Work out the finished part from the listing and answer in its coordinate system (mm). A direction names the side the tool comes from. Coordinates: 2 decimals unless noted, no trailing zeros. Loops run counter-clockwise (first coordinate to the right, second up) from the corner with the lowest first, then second, coordinate; pieces in that order, holes last. Notation, with made-up numbers: (65.25, 59) - (81.25, 59) arc R36 ccw to (81.25, 97) - close; hole circle Ø11 at (53, 28.5). An arc over 180 degrees is marked (long way). Write each question's results on one line, items separated by ' | '. Start each with the question number.
1. A cutting plane is placed at B-B on x = 0. Determine the outline of the cut face in (y, z), then the cut area to 3 significant figures.
2. A cutting plane is placed at C-C on z = 37.5. Determine the outline of the cut face in (x, y).
3. Determine the mould class of faces 1 (the cylindrical face through (-1.319, -7.395, -59.985)), 2 (the cylindrical face through (-2.17, -7.4, 20.24)), 3 (the cylindrical face through (-2.17, -7.4, -9.76)), 4 (the cylindrical face through (22.985, -7.605, 2.852)) for opening direction X: released by +X, released by -X, zero draft, split by the parting line, or undercut.
4. Which of the six approach directions +Z, -Z, +X, -X, +Y, -Y give full straight-line access (tool end or side, diameter ignored) to faces 5 (the flat face through (-45, -7, 0)), 6 (the flat face through (-1, 0, -16)), 7 (the flat face through (45, -7, 0))?
5. A cutting plane is placed at D-D on z = 25. Determine the outline of the cut face in (x, y), then the cut area to 3 significant figures.
6. Each of these flat-tipped pins is pushed along its axis until it touches: P1, Ø3, axis at x = -16, y = -7.5, coming from the -Z side; P2, Ø1.5, axis at x = -45.5, y = -12.5, coming from the +Z side; P3, Ø4.5, axis at y = -9.5, z = 18, coming from the +X side. Where does it stop, or does it pass through?
7. A cutting plane is placed at A-A on y = -3. Determine the outline of the cut face in (x, z).
8. Find the intervals of material crossed by line 1 along Z through (x, y) = (0, -4.75); line 2 along Z through (x, y) = (-4, -4.75); line 3 along X through (y, z) = (-9.5, 36.5), in increasing order. Write a range as [from, to].
from build123d import *

# Parameters (mm, degrees)
F0_R     = 10
F1_DEPTH = 15
F2_R     = 10
F3_R     = 10


with BuildPart() as f1:
    # F0 (on Front) → F1 (new body)
    with BuildSketch(Plane.XZ):
        with BuildLine():
            Line((-19.702956, 0), (-60, 0))
            ThreePointArc((-60, 0), (0, -60), (60, 0))
            Line((60, 0), (19.977827, 0))
            Line((19.977827, 0), (19.977827, 29.058505))
            ThreePointArc((19.977827, 29.058505), (0.37156, 49.996548), (-19.999013, 29.801323))
            Line((-19.999013, 29.801323), (-19.702956, 0))
        make_face()
        Circle(F0_R, mode=Mode.SUBTRACT)
        with Locations((0, 30)):
            Circle(F0_R, mode=Mode.SUBTRACT)
    extrude(amount=F1_DEPTH)

    # F2
    f2_edges = [f1.edges().sort_by_distance(p)[0] for p in [
        (19.977827, -7.5, 0),
    ]]
    fillet(f2_edges, radius=F2_R)

    # F3
    f3_edges = [f1.edges().sort_by_distance(p)[0] for p in [
        (-19.702956, -7.5, 0),
    ]]
    fillet(f3_edges, radius=F3_R)


solid = f1.part
Values:
1) outline: (-15, -60) - (0, -60) - (0, -10) - (-15, -10) - close; (-15, 10) - (0, 10) - (0, 20) - (-15, 20) - close; (-15, 40) - (0, 40) - (0, 50) - (-15, 50) - close | area: 1,050 mm^2
2) outline: (-18.54, -15) - (-6.61, -15) - (-6.61, 0) - (-18.54, 0) - close; (6.61, -15) - (18.54, -15) - (18.54, 0) - (6.61, 0) - close
3) face 1: split by the parting line | face 2: undercut | face 3: undercut | face 4: released by +X
4) face 5: +Z, -X, +Y, -Y | face 6: +Z, -Z, +X, -X, +Y | face 7: +Z, +X, +Y, -Y
5) outline: (-19.95, -15) - (-8.66, -15) - (-8.66, 0) - (-19.95, 0) - close; (8.66, -15) - (19.98, -15) - (19.98, 0) - (8.66, 0) - close | area: 339 mm^2
6) P1: z = -58.22 | P2: z = 0 | P3: x = 19.98
7) outline: (-60, 0) arc R60 ccw to (60, 0) - (29.98, 0) arc R10 cw to (19.98, 10) - (19.98, 29.06) arc R20 ccw (long way) to (-20, 29.8) - (-19.8, 10.1) arc R10 cw to (-29.8, 0) - close; hole circle Ø20 at (0, 0); hole circle Ø20 at (0, 30)
8) line 1: [-60, -10], [10, 20], [40, 50] | line 2: [-59.87, -9.17], [9.17, 20.83], [39.17, 49.6] | line 3: [-18.91, -7.6], [7.6, 18.91]
